Verification items for the finished model (mm, model axes). A direction names the side the tool comes from. Round coordinates to 2 decimals unless told otherwise and drop trailing zeros. Write each loop counter-clockwise with the first axis right and the second up, starting at its lowest first coordinate (ties: lowest second). Pieces come first, ordered by that corner, then holes. Notation, with made-up numbers: M 13.5,2.25 L 67.5,2.25 A15 ccw 67.5,20.25 Z; hole C -10.75,87.5 d3. An arc over 180 degrees is marked long. Answer in a Markdown table with one row per item. Add a question column.
1. Sectioned sample at D-D on x = 71.5. Record the cut outline in (y, z).
2. Set-up check for faces 1 (the flat face through (-93.53, -14.79, 341.05)), 2 (the flat face through (199, -15, 0)): record each of +Z, -Z, +X, -X, +Y, -Y from which the full face is reachable in a straight line by a thin tool's end or side.
3. Sectioned sample at A-A on y = -9.75. Record the cut outline in (x, z), plus the area to 3 significant figures.
4. Draft check along Z on faces 3 (the cylindrical face through (-15.48, -14.79, 764.19)), 4 (the flat face through (-80, 0, 418)), 5 (the flat face through (90.947, -14.79, 350.735)), 6 (the cylindrical face through (0.783, -14.79, 774.988)). Enter one of: pulls with the +Z half, pulls with the -Z half, needs draft (parallel to the pull), parting line crosses it, or undercut.
5. Go/stop test with flat-tipped pins: pin 1 Ø2 at (y, z) = (-18.5, 309.5) entering from -X; pin 2 Ø8 at (y, z) = (-19.5, 535) entering from +X; pin 3 Ø8 at (x, z) = (77, 388) entering from -Y; pin 4 Ø1.5 at (y, z) = (-17.5, 324) entering from -X. Record where each tip stops, or that it passes through.
6. Sectioned sample at C-C on z = 602.5. Record the cut outline in (x, y).
7. Material ranges on probe 1 along X at (y, z) = (-12.5, 611.5); probe 2 along X at (y, z) = (-2.5, 60.5), recorded low to high.
8. Sectioned sample at B-B on z = 750. Record the cut outline in (x, y), plus the area to 3 significant figures.
```python
from build123d import *

# Parameters (mm, degrees)
F0_R     = 21
F1_DEPTH = 30


with BuildPart() as f1:
    # F0 (on Front) → F1 (new body)
    with BuildSketch(Plane.XZ):
        with BuildLine():
            Line((20.93509, 729.709066), (19.646777, 734.540241))
            ThreePointArc((19.646777, 734.540241), (15, 730), (9.340271, 726.810361))
            Line((9.340271, 726.810361), (8.051958, 721.979187))
            Line((8.051958, 721.979187), (0, 691.784345))
            Line((0, 691.784345), (184.475825, 0))
            Line((184.475825, 0), (213.462873, 0))
            Line((213.462873, 0), (213.462873, 7.72988))
            Line((213.462873, 7.72988), (20.93509, 729.709066))
        make_face()
        with BuildLine():
            Line((-20.93509, 729.709066), (-213.462873, 7.72988))
            Line((-213.462873, 7.72988), (-213.462873, 0))
            Line((-213.462873, 0), (-184.475825, 0))
            Line((-184.475825, 0), (0, 691.784345))
            Line((0, 691.784345), (-8.051958, 721.979187))
            Line((-8.051958, 721.979187), (-9.340271, 726.810361))
            ThreePointArc((-9.340271, 726.810361), (-15, 730), (-19.646777, 734.540241))
            Line((-19.646777, 734.540241), (-20.93509, 729.709066))
        make_face()
        with BuildLine():
            ThreePointArc((19.646777, 734.540241), (0, 775), (-19.646777, 734.540241))
            ThreePointArc((-19.646777, 734.540241), (-15, 730), (-9.340271, 726.810361))
            Line((-9.340271, 726.810361), (-8.051958, 721.979187))
            Line((-8.051958, 721.979187), (0, 691.784345))
            Line((0, 691.784345), (8.051958, 721.979187))
            Line((8.051958, 721.979187), (9.340271, 726.810361))
            ThreePointArc((9.340271, 726.810361), (15, 730), (19.646777, 734.540241))
        make_face()
        with Locations((0, 750)):
            Circle(F0_R, mode=Mode.SUBTRACT)
    extrude(amount=F1_DEPTH)


solid = f1.part
```
Geometry check:
| question | item | result |
|---|---|---|
| 1 | outline | M -30,423.66 L 0,423.66 L 0,540.09 L -30,540.09 Z |
| 2 | face 1 | -Z, +Y, -Y |
| 2 | face 2 | -Z, +X, -X, +Y, -Y |
| 3 | outline | M -213.46,0 L -184.48,0 L 0,691.78 L 184.48,0 L 213.46,0 L 213.46,7.73 L 19.65,734.54 A25 ccw long -19.65,734.54 L -213.46,7.73 Z; hole C 0,750 d42 |
| 3 | area | 45,400 mm2 |
| 4 | face 3 | undercut |
| 4 | face 4 | needs draft |
| 4 | face 5 | pulls with the -Z half |
| 4 | face 6 | undercut |
| 5 | pin 1 | stops at x = -133.26 |
| 5 | pin 2 | stops at x = 73.92 |
| 5 | pin 3 | stops at y = -30 |
| 5 | pin 4 | stops at x = -129.32 |
| 6 | outline | M -54.86,-30 L -23.81,-30 L -23.81,0 L -54.86,0 Z; M 23.81,-30 L 54.86,-30 L 54.86,0 L 23.81,0 Z |
| 7 | probe 1 | x = -52.46 to -21.41, 21.41 to 52.46 |
| 7 | probe 2 | x = -199.39 to -168.34, 168.34 to 199.39 |
| 8 | outline | M -25,-30 L -21,-30 L -21,0 L -25,0 Z; M 21,-30 L 25,-30 L 25,0 L 21,0 Z |
| 8 | area | 240 mm2 |
